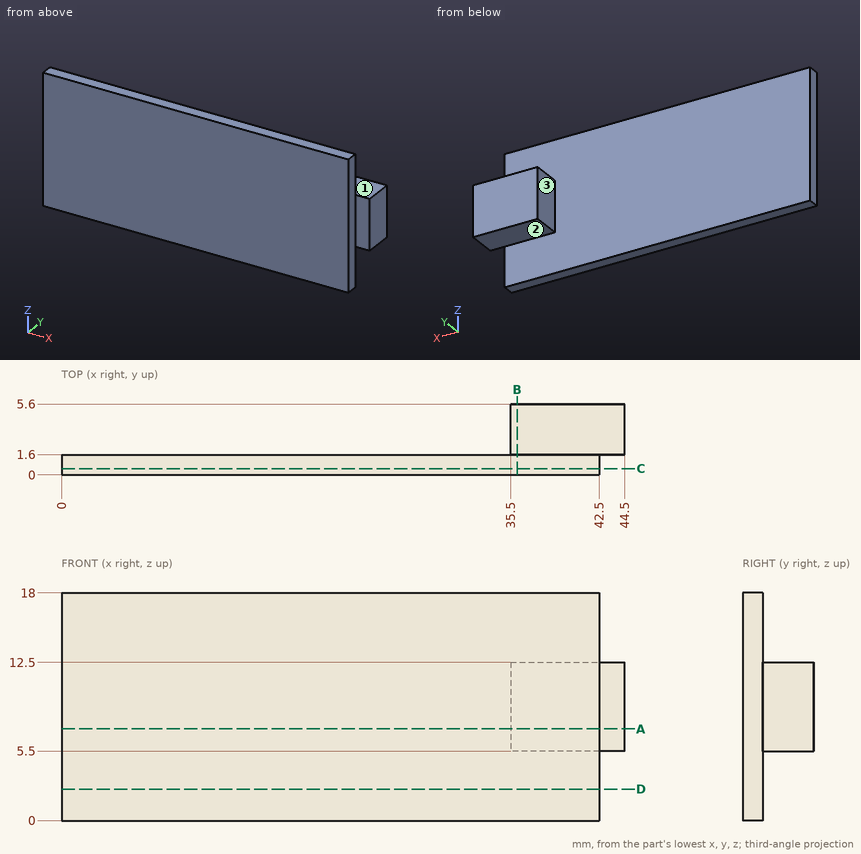
Could you check a few things on this drawing? It's one solid part, dimensions in mm from its lowest x, y, z. A direction names the side the tool comes from. Give positions to 0.01 mm unless a question says otherwise; leave off trailing zeros. Order: outer loops, then holes, each group sorted by start corner. A loop starts at its lowest first (then second) coordinate and runs counter-clockwise, first axis right, second up. Notation, with made-up numbers: (27, 5.25) -> (56, 5.25) arc R24 ccw to (56, 39.25) -> close; hole circle Ø10 at (-15, -33.5). An arc over 180 degrees is marked (long way). Answer in a Markdown table with one row per item. Add a question column.
Item 1: Imagine slicing it at D-D (z = 2.5). List the corners of the cut face in (x, y) for me, and give its area (3 significant figures).
Item 2: Please list where these lines run through material, in increasing order: probe 1 along Z at (x, y) = (37, 2); probe 2 along Y at (x, z) = (30.5, 14); probe 3 along X at (y, z) = (3.85, 10).
Item 3: Imagine slicing it at A-A (z = 7.25). List the corners of the cut face in (x, y) for me, and give its area (3 significant figures).
Item 4: Imagine slicing it at C-C (y = 0.5). List the corners of the cut face in (x, z) for me.
Item 5: I'm going to push flat-ended pins straight in: P1, Ø1, axis at x = 9.5, y = 4, coming from the -Z side; P2, Ø3, axis at x = 38, y = 4, coming from the +Z side; P3, Ø1.8, axis at y = 0.5, z = 9, coming from the +X side; P4, Ø1.2, axis at y = 3.5, z = 10.5, coming from the -X side. Where does each tip first touch, or does it pass through?
Item 6: Imagine slicing it at B-B (x = 36). List the corners of the cut face in (y, z) for me, and give its area (3 significant figures).
Item 7: For the marked faces 1, 2 and 3, which set-ups out of +Z, -Z, +X, -X, +Y, -Y let a thin tool reach every point of the face, with its end or its side?
Result:
| question | item | result |
|---|---|---|
| 1 | outline | (0, 0) -> (42.5, 0) -> (42.5, 1.6) -> (0, 1.6) -> close |
| 1 | area | 68.0 mm2 |
| 2 | probe 1 | 5.5 to 12.5 |
| 2 | probe 2 | 0 to 1.6 |
| 2 | probe 3 | 35.5 to 44.5 |
| 3 | outline | (0, 0) -> (42.5, 0) -> (42.5, 1.6) -> (44.5, 1.6) -> (44.5, 5.6) -> (35.5, 5.6) -> (35.5, 1.6) -> (0, 1.6) -> close |
| 3 | area | 104 mm2 |
| 4 | outline | (0, 0) -> (42.5, 0) -> (42.5, 18) -> (0, 18) -> close |
| 5 | P1 | through |
| 5 | P2 | z = 12.5 |
| 5 | P3 | x = 42.5 |
| 5 | P4 | x = 35.5 |
| 6 | outline | (0, 0) -> (1.6, 0) -> (1.6, 5.5) -> (5.6, 5.5) -> (5.6, 12.5) -> (1.6, 12.5) -> (1.6, 18) -> (0, 18) -> close |
| 6 | area | 56.8 mm2 |
| 7 | face 1 | +Z, +X, -X, +Y |
| 7 | face 2 | -Z, +X, -X, +Y |
| 7 | face 3 | +Z, -Z, -X, +Y |
